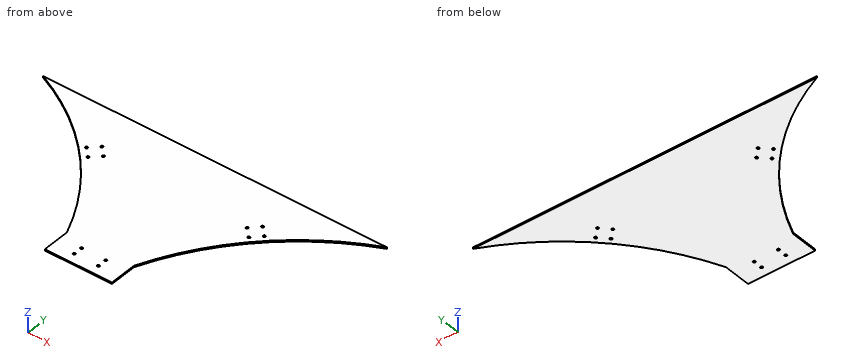
Autodesk Inventor part; units mm, degrees
ref_plane "YZ Plane" through (0, 0, 0) normal (1, 0, 0) x (0, 1, 0)
ref_plane "XZ Plane" through (0, 0, 0) normal (0, 1, 0) x (-1, 0, 0)
ref_plane "XY Plane" through (0, 0, 0) normal (0, 0, 1) x (1, 0, 0)
sketch "Sketch1" plane through (0, 0, 0) normal (0, 0, 1) x (1, 0, 0)
  line L0 (70.485, -28.575) -> (-70.485, -28.575)
  line L1 (-70.485, -28.575) -> (-70.485, 28.575)
  line L2 (-70.485, 28.575) -> (70.485, 28.575)
  line L3 (70.485, 28.575) -> (70.485, -28.575)
  line L4 (70.485, -28.575) -> (-70.485, 28.575) construction
  line L5 (-70.485, -28.575) -> (70.485, 28.575) construction
  line L6 (-361.95, 327.025) -> (361.95, 327.025)
  line L7 (-361.95, 327.025) -> (-361.95, 352.425) construction
  line L8 (-70.485, 28.575) -> (-45.085, 28.575) construction
  line L9 (0, 0) -> (0, 28.575) construction
  arc A0 (-70.485, 28.575) -> (-361.95, 327.025) centre (-587.1049, -184.407) ccw
  arc A1 (361.95, 327.025) -> (70.485, 28.575) centre (587.1049, -184.407) ccw
  point P0 (0, 327.025)
  dimension "d0" = 140.97
  dimension "d1" = 57.15
  dimension "d2" = 723.9
  dimension "d3" = 355.6
  dimension "d4" = 25.4
  dimension "d7" = 558.8
extrude "Plate1" add sketch "Sketch1" along normal blind 3.048
sketch "Sketch2" plane through (0, 0, 3.048) normal (0, 0, 1) x (1, 0, 0)
  line L0 (70.485, -28.575) -> (-70.485, -28.575) construction
  line L1 (-25.4, -28.575) -> (-25.4, -7.9375) construction
  point P0 (0, 0)
  point P1 (25.4, -7.9375)
  point P2 (-25.4, 11.1125)
  point P3 (25.4, 11.1125)
  dimension "d9" = 20.6375
  dimension "d11" = 25.4
  dimension "d15" = 50.8
  dimension "d18" = 19.05
hole "Hole1" at (-25.4, -7.9375, 3.048) at (25.4, -7.9375, 3.048) at (-25.4, 11.1125, 3.048) at (25.4, 11.1125, 3.048) direction (0, 0, -1) diameter 5.1054 depth 3.048 tip angle 118
sketch "Sketch3" plane through (0, 0, 0) normal (0, 0, -1) x (-1, 0, 0)
  arc A0 (361.95, 327.025) -> (70.485, 28.575) centre (587.1049, -184.407) ccw construction
  line L0 (187.323, 206.0182) -> (178.2371, 214.8915) construction
  line L1 (169.3637, 205.8056) -> (187.1104, 223.9775) construction
  line L2 (169.3637, 205.8056) -> (151.1918, 223.5522) construction
  line L3 (187.1104, 223.9775) -> (168.9384, 241.7241) construction
  line L4 (0, 0) -> (0, 25.4) construction
  point P0 (-169.3637, 205.8056)
  point P1 (-187.1104, 223.9775)
  point P2 (-151.1918, 223.5522)
  point P3 (-168.9384, 241.7241)
  dimension "d28" = 12.7
  dimension "d29" = 25.4
  dimension "d30" = 25.4
  dimension "d31" = 25.4
  dimension "d32" = 25.4
hole "Hole2" at (-169.3637, 205.8056, 0) at (-187.1104, 223.9775, 0) at (-151.1918, 223.5522, 0) at (-168.9384, 241.7241, 0) at (151.1918, 223.5522, 0) at (169.3637, 205.8056, 0) at (187.1104, 223.9775, 0) at (168.9384, 241.7241, 0) direction (0, 0, 1) diameter 5.1054 depth 3.048 tip angle 118
sketch "Sketch4" plane through (0, 0, 0) normal (0, 0, -1) x (-1, 0, 0)
  point P0 (0, 0)
equation "\"d26\" = Thickness"
equation "\"d38\" = Thickness"
equation "\"d8\" = Thickness"
equation "\"BendRadius\" = Thickness"
equation "\"BendReliefWidth\" = Thickness"
equation "\"BendReliefDepth\" = 0.5 * Thickness"
equation "\"CornerReliefSize\" = 4 * Thickness"
equation "\"MinimumRemnant\" = 2 * Thickness"
equation "\"TransitionRadius\" = BendRadius"
equation "\"JacobiRadiusSize\" = BendRadius"
equation "\"GapSize\" = Thickness"
properties part number "curved_hopper_back" material "Polycarbonate, Clear"
Read the model definition and answer for the solid it produces. Units are mm, in the model's axes. Round coordinates to 2 decimals unless told otherwise and drop trailing zeros. Write each loop counter-clockwise with the first axis right and the second up, starting at its lowest first coordinate (ties: lowest second). Pieces come first, ordered by that corner, then holes.
Q1. Straight lines are drawn through the part: line 1 (X direction, y = 11.5, z = 2.1) (3 decimals); line 2 (Y direction, x = -25.4, z = 1.6) (3 decimals); line 3 (X direction, y = -4.5, z = 2.95) (3 decimals). For each, find the intervals that lie inside material, in ascending order.
Values:
line 1: x = -70.485 to -27.923, -22.877 to 22.877, 27.923 to 70.485
line 2: y = -28.575 to -10.49, -5.385 to 8.56, 13.665 to 327.025
line 3: x = -70.485 to 70.485
Q2. Find section B-B on y = 186.5. Determine the outline of the cut face in (x, z), and give its area (3 significant figures).
Values:
outline: (-169.15, 0) - (169.15, 0) - (169.15, 3.05) - (-169.15, 3.05) - close
area: 1,030 mm2
Q3. Flat-ended cylindrical pins translate along their axes: P1, Ø1, axis at y = 18, z = 0.5, coming from the +X side (3 decimals); P2, Ø1, axis at x = -162.5, z = 2, coming from the -Y side; P3, Ø0.9, axis at y = -14.5, z = 2, coming from the -X side (3 decimals). Find the tip coordinate at first contact, or state that the pin passes through.
Values:
P1: stops at x = 70.485
P2: stops at y = 178.28
P3: stops at x = -70.485
Q4. Find section C-C on x = -264.5. Determine the outline of the cut face in (y, z) (3 decimals).
Values:
outline: (271.864, 0) - (327.025, 0) - (327.025, 3.048) - (271.864, 3.048) - close
Q5. Find section A-A on z = 2.55. State how many separate pieces and enclosed holes the cut face has, and give its area (3 significant figures).
Values:
separate pieces: 1
enclosed holes: 12
area: 114,000 mm2
